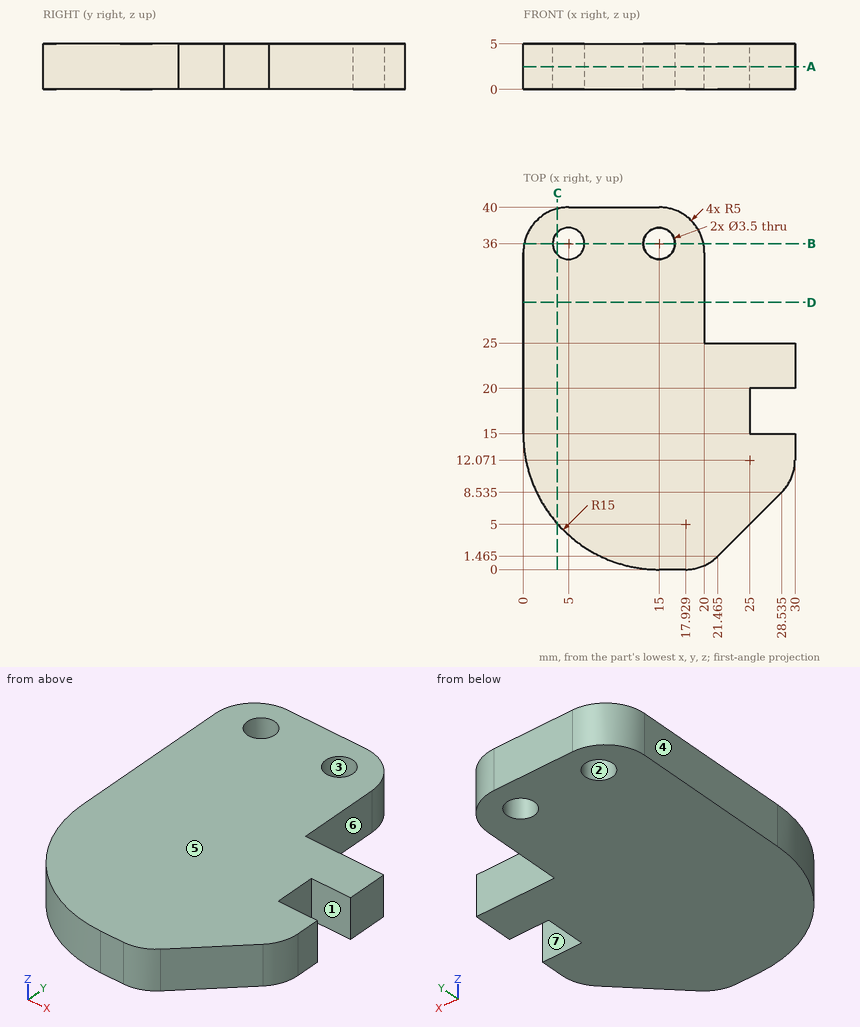
Check sheet for the drawn part. Datum: minimum x, y, z corner. Units: mm. A direction names the side the tool comes from. Round coordinates to 2 decimals unless told otherwise and drop trailing zeros. Loops run counter-clockwise (first coordinate to the right, second up) from the corner with the lowest first, then second, coordinate; pieces in that order, holes last.
Item 1: Cross-section at D-D on y = 29.5. Record the boundary of the cut face in (x, z).
Item 2: Mould release check, pull along X, two halves, no side actions. Record for the marked faces 1, 2, 3 and 4: pulls with the +X half, pulls with the -X half, needs draft (parallel to the pull), parting line crosses it, or undercut.
Item 3: Cross-section at C-C on x = 3.75. Record the boundary of the cut face in (y, z) (1 decimal).
Item 4: Access from +Z, -Z, +X, -X, +Y, -Y to the whole of each face (thin tool, end or side, straight path). Record for the marked faces 5, 6 and 7.
Item 5: Thickness scan on line 1 (Y direction, x = 15, z = 1.15); line 2 (Y direction, x = 5, z = 1.4); line 3 (X direction, y = 16.5, z = 2.9). Record the ranges inside material, lowest first.
Item 6: Cross-section at B-B on y = 36. Record the boundary of the cut face in (x, z).
Item 7: Cross-section at A-A on z = 2.5. Count the separate pieces of the cut face and the enclosed holes in it, then the cut area to 3 significant figures.
Item 8: Gauge pin test, flat ends, axial feed: pin 1 (2.5 mm diameter, centred on x = 24.5, z = 1.5, fed in from +Y); pin 2 (1 mm diameter, centred on y = 10, z = 4, fed in from -X); pin 3 (2.5 mm diameter, centred on y = 18.5, z = 1.5, fed in from +X). Record the tip position at first contact, or that the pin passes through.
Answer sheet:
1. outline: (0, 0) - (20, 0) - (20, 5) - (0, 5) - close
2. face 1: needs draft
2. face 2: undercut
2. face 3: undercut
2. face 4: pulls with the -X half
3. outline: (5.1, 0) - (34.8, 0) - (34.8, 5) - (5.1, 5) - close; (37.2, 0) - (39.8, 0) - (39.8, 5) - (37.2, 5) - close
4. face 5: +Z, +X, -X, +Y, -Y
4. face 6: +Z, -Z, +X, +Y
4. face 7: +Z, -Z, +X
5. line 1: y = 0 to 34.25, 37.75 to 40
5. line 2: y = 3.82 to 34.25, 37.75 to 40
5. line 3: x = 0 to 25
6. outline: (0.1, 0) - (3.25, 0) - (3.25, 5) - (0.1, 5) - close; (6.75, 0) - (13.25, 0) - (13.25, 5) - (6.75, 5) - close; (16.75, 0) - (19.9, 0) - (19.9, 5) - (16.75, 5) - close
7. separate pieces: 1
7. enclosed holes: 2
7. area: 896 mm2
8. pin 1: stops at y = 25
8. pin 2: stops at x = 0.69
8. pin 3: stops at x = 25
